from build123d import *

# Parameters (mm, degrees)
F0_R     = 13.954927
F1_DEPTH = 2
F2_R     = 5.95
F2_R_2   = 3.95
F3_DEPTH = 2
F2_R_3   = 8.45
F2_R_4   = 6.95
F4_DEPTH = 2


with BuildPart() as f1:
    # F0 (on Top) → F1 (new body)
    with BuildSketch(Plane.XY):
        Circle(F0_R)
    extrude(amount=F1_DEPTH)

    # F2 (on face) → F3 (join)
    with BuildSketch(Plane.XY.offset(2)):
        Circle(F2_R)
        Circle(F2_R_2, mode=Mode.SUBTRACT)
    extrude(amount=F3_DEPTH)

    # F2 (on face) → F4 (join)
    with BuildSketch(Plane.XY.offset(2)):
        Circle(F2_R_3)
        Circle(F2_R_4, mode=Mode.SUBTRACT)
    extrude(amount=F4_DEPTH)


solid = f1.part
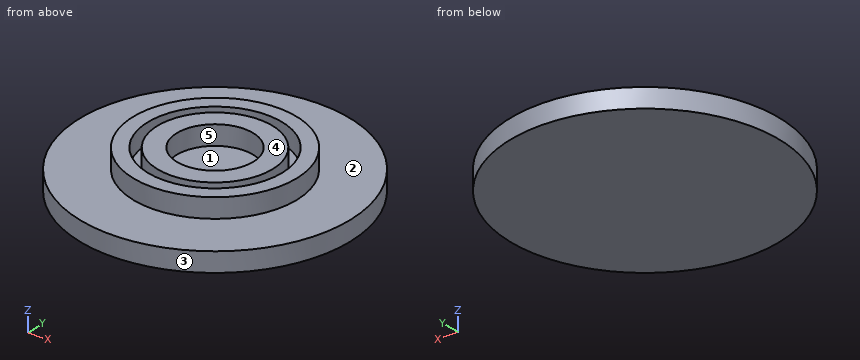
Geometry check sheet. Reference: the model listing, model coordinates, mm. Face numbers are marked on the shaded views. A direction names the side the tool comes from. Round coordinates to 2 decimals unless told otherwise and drop trailing zeros. Order: outer loops, then holes, each group sorted by start corner. A loop starts at its lowest first (then second) coordinate and runs counter-clockwise, first axis right, second up. Notation, with made-up numbers: (50, 1.25) - (95, 1.25) arc R20 ccw to (95, 33.25) - close; hole circle Ø11 at (-12.75, 79.5). An arc over 180 degrees is marked (long way). One line per question, with ' | ' between items. Start each with the question number.
(1) Depth check by flat-ended pin: pin 1 Ø7 at (x, y) = (0, 0) entering from +Z; pin 2 Ø8 at (x, y) = (11, -9) entering from -Z. Enter the tip coordinate at first touch or a pass-through.
(2) Release check for a two-part mould opening along X. For the marked faces 1, 2 and 3 record: released by +X, released by -X, zero draft, split by the parting line, or undercut.
(3) Sectioned sample at D-D on x = -10.5. Record the cut outline in (y, z), and give its area (3 significant figures).
(4) Sectioned sample at C-C on y = -7.5. Record the cut outline in (x, z).
(5) Thickness scan on L1, parallel to Y at x = 0, z = 2.5; L2, parallel to Y at x = 4.5, z = 2.05; L3, parallel to Z at x = -6.75, y = -7.5. Record the ranges inside material, lowest first. Write a range as [from, to].
(6) Sectioned sample at A-A on x = 0. Record the cut outline in (y, z), and give its area (3 significant figures).
(7) Access from +Z, -Z, +X, -X, +Y, -Y to the whole of each face (thin tool, end or side, straight path). Record for the marked faces 4 and 5.
Conclusion:
1) pin 1: stops at z = 2 | pin 2: stops at z = 0
2) face 1: undercut | face 2: zero draft | face 3: split by the parting line
3) outline: (-9.19, 0) - (9.19, 0) - (9.19, 2) - (-9.19, 2) - close | area: 36.8 mm2
4) outline: (-11.77, 0) - (11.77, 0) - (11.77, 2) - (3.89, 2) - (3.89, 4) - (-3.89, 4) - (-3.89, 2) - (-11.77, 2) - close
5) L1: y = [-8.45, -6.95], [-5.95, -3.95], [3.95, 5.95], [6.95, 8.45] | L2: y = [-7.15, -5.3], [-3.89, 3.89], [5.3, 7.15] | L3: z = [0, 2]
6) outline: (-13.95, 0) - (13.95, 0) - (13.95, 2) - (8.45, 2) - (8.45, 4) - (6.95, 4) - (6.95, 2) - (5.95, 2) - (5.95, 4) - (3.95, 4) - (3.95, 2) - (-3.95, 2) - (-3.95, 4) - (-5.95, 4) - (-5.95, 2) - (-6.95, 2) - (-6.95, 4) - (-8.45, 4) - (-8.45, 2) - (-13.95, 2) - close | area: 69.8 mm2
7) face 4: +Z, +X, -X, +Y, -Y | face 5: +Z
